```python
from build123d import *

# Parameters (mm, degrees)
SKETCH2_R           = 100
BOSS_EXTRUDE1_DEPTH = 5
CUT_EXTRUDE2_DEPTH  = 5


with BuildPart() as part:
    # Sketch2 → Boss-Extrude1 (new body)
    with BuildSketch(Plane(origin=(0, 0, 0), x_dir=(1, 0, 0), z_dir=(0, 1, 0))):
        Circle(SKETCH2_R)
        with BuildLine():
            Line((-8, -12.68857754), (-8, -84.622691992))
            ThreePointArc((-8, -84.622691992), (-60.104076401, -60.104076401), (-84.622691992, -8))
            Line((-84.622691992, -8), (-12.68857754, -8))
            ThreePointArc((-12.68857754, -8), (-10.606601718, -10.606601718), (-8, -12.68857754))
        make_face(mode=Mode.SUBTRACT)
        with BuildLine():
            Line((12.68857754, -8), (84.622691992, -8))
            ThreePointArc((84.622691992, -8), (60.104076401, -60.104076401), (8, -84.622691992))
            Line((8, -84.622691992), (8, -12.68857754))
            ThreePointArc((8, -12.68857754), (10.606601718, -10.606601718), (12.68857754, -8))
        make_face(mode=Mode.SUBTRACT)
        with BuildLine():
            Line((-8, 84.622691992), (-8, 12.68857754))
            ThreePointArc((-8, 12.68857754), (-10.606601718, 10.606601718), (-12.68857754, 8))
            Line((-12.68857754, 8), (-84.622691992, 8))
            ThreePointArc((-84.622691992, 8), (-60.104076401, 60.104076401), (-8, 84.622691992))
        make_face(mode=Mode.SUBTRACT)
        with BuildLine():
            ThreePointArc((8, 84.622691992), (60.104076401, 60.104076401), (84.622691992, 8))
            Line((84.622691992, 8), (12.68857754, 8))
            ThreePointArc((12.68857754, 8), (10.606601718, 10.606601718), (8, 12.68857754))
            Line((8, 12.68857754), (8, 84.622691992))
        make_face(mode=Mode.SUBTRACT)
    extrude(amount=BOSS_EXTRUDE1_DEPTH)

    # Sketch3 → Cut-Extrude2 (cut)
    with BuildSketch(Plane.XZ):
        with BuildLine():
            Line((1.5, 0), (1.5, -1.322875656))
            ThreePointArc((1.5, -1.322875656), (-2, 0), (1.5, 1.322875656))
            Line((1.5, 1.322875656), (1.5, 0))
        make_face()
    extrude(amount=-CUT_EXTRUDE2_DEPTH, mode=Mode.SUBTRACT)


solid = part.part
```
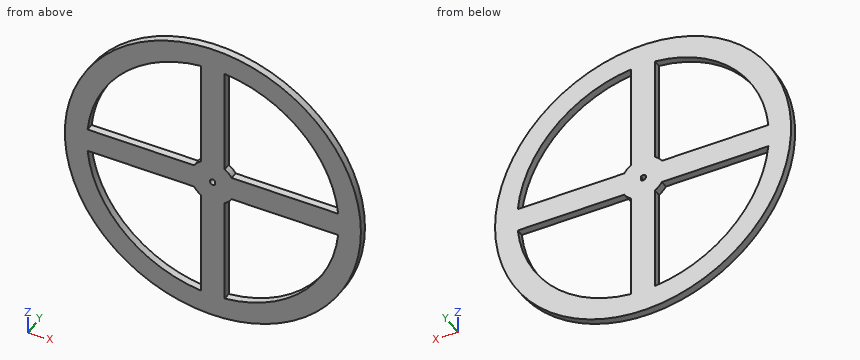
Geometry check sheet. Reference: the model listing, model coordinates, mm. Coordinates: 2 decimals unless noted, no trailing zeros. Order: outer loops, then holes, each group sorted by start corner. A loop starts at its lowest first (then second) coordinate and runs counter-clockwise, first axis right, second up.
Item 1: Section check C-C (z = -36). Enter the section's corners in (x, y), plus the area to 3 significant figures.
Item 2: Scan lines: line 1 along X through (y, z) = (3.2, 0); line 2 along Z through (x, y) = (0, 1.45); line 3 along Z through (x, y) = (-11.5, 2.45). Record each from-to range of solid material in increasing order.
Item 3: Section check B-B (x = 82). Enter the section's corners in (y, z).
Item 4: Depth check by flat-ended pin: pin 1 (1.5 mm diameter, centred on y = 3.5, z = -46.5, fed in from +X); pin 2 (2.5 mm diameter, centred on y = 2.5, z = 59, fed in from +X); pin 3 (2.5 mm diameter, centred on x = -63, y = 2, fed in from -Z). Enter the tip coordinate at first touch or a pass-through.
Item 5: Section check A-A (y = 2). Enter the section's corners in (x, z).
Check sheet entries:
1. outline: (-93.3, 0) - (-77, 0) - (-77, 5) - (-93.3, 5) - close; (-8, 0) - (8, 0) - (8, 5) - (-8, 5) - close; (77, 0) - (93.3, 0) - (93.3, 5) - (77, 5) - close
1. area: 243 mm2
2. line 1: x = -100 to -2, 1.5 to 100
2. line 2: z = -100 to -2, 2 to 100
2. line 3: z = -99.34 to -84.22, -9.63 to 9.63, 84.22 to 99.34
3. outline: (0, -57.24) - (5, -57.24) - (5, -22.38) - (0, -22.38) - close; (0, -8) - (5, -8) - (5, 8) - (0, 8) - close; (0, 22.38) - (5, 22.38) - (5, 57.24) - (0, 57.24) - close
4. pin 1: stops at x = 88.92
4. pin 2: stops at x = 81.64
4. pin 3: stops at z = -78.66
5. outline: circle Ø200 at (0, 0); hole (-84.62, -8) arc R85 ccw to (-8, -84.62) - (-8, -12.69) arc R15 cw to (-12.69, -8) - close; hole (-84.62, 8) - (-12.69, 8) arc R15 cw to (-8, 12.69) - (-8, 84.62) arc R85 ccw to start; hole (1.5, -1.32) - (1.5, 1.32) arc R2 ccw (long way) to start; hole (8, -84.62) arc R85 ccw to (84.62, -8) - (12.69, -8) arc R15 cw to (8, -12.69) - close; hole (8, 12.69) arc R15 cw to (12.69, 8) - (84.62, 8) arc R85 ccw to (8, 84.62) - close
